Verification items for this drawing (mm, ordinates from the low corner). A direction names the side the tool comes from. Give positions to 0.01 mm unless a question says otherwise; leave off trailing zeros. Write each loop counter-clockwise with the first axis right and the second up, starting at its lowest first coordinate (ties: lowest second). Pieces come first, ordered by that corner, then holes. Notation, with made-up numbers: (49, 55.25) -> (65, 55.25) arc R27 cw to (65, 86.25) -> close; hole circle Ø6 at (20, 14.25). An arc over 180 degrees is marked (long way). Use one line per item in the form item = value. Start each with the question number.
(1) Section check A-A, the plane z = 19.25. Record the cut outline in (x, y).
(2) Section check B-B, the plane y = 9.75. Record the cut outline in (x, z).
(3) Section check C-C, the plane x = 4. Record the cut outline in (y, z), plus the area to 3 significant figures.
(4) Scan lines: L1, parallel to Z at x = 7, y = 0.5; L2, parallel to Z at x = 5.75, y = 12 (1 decimal); L3, parallel to Z at x = 7, y = 5.5. Record each from-to range of solid material in increasing order.
(5) Depth check by flat-ended pin: pin 1 Ø1 at (y, z) = (4, 7) entering from -X; pin 2 Ø7 at (x, y) = (6.57, 6.9) entering from +Z; pin 3 Ø6 at (y, z) = (10.5, 17) entering from -X. Enter the tip coordinate at first touch or a pass-through.
(6) Section check D-D, the plane y = 6.9. Record the cut outline in (x, z) (1 decimal).
(7) Set-up check for the marked faces 1, 2 and 3: record each of +Z, -Z, +X, -X, +Y, -Y from which the full face is reachable in a straight line by a thin tool's end or side.
(8) Release check for a two-part mould opening along Z. For the marked faces 4, 5 and 6 record: pulls with the +Z half, pulls with the -Z half, needs draft (parallel to the pull), parting line crosses it, or undercut.
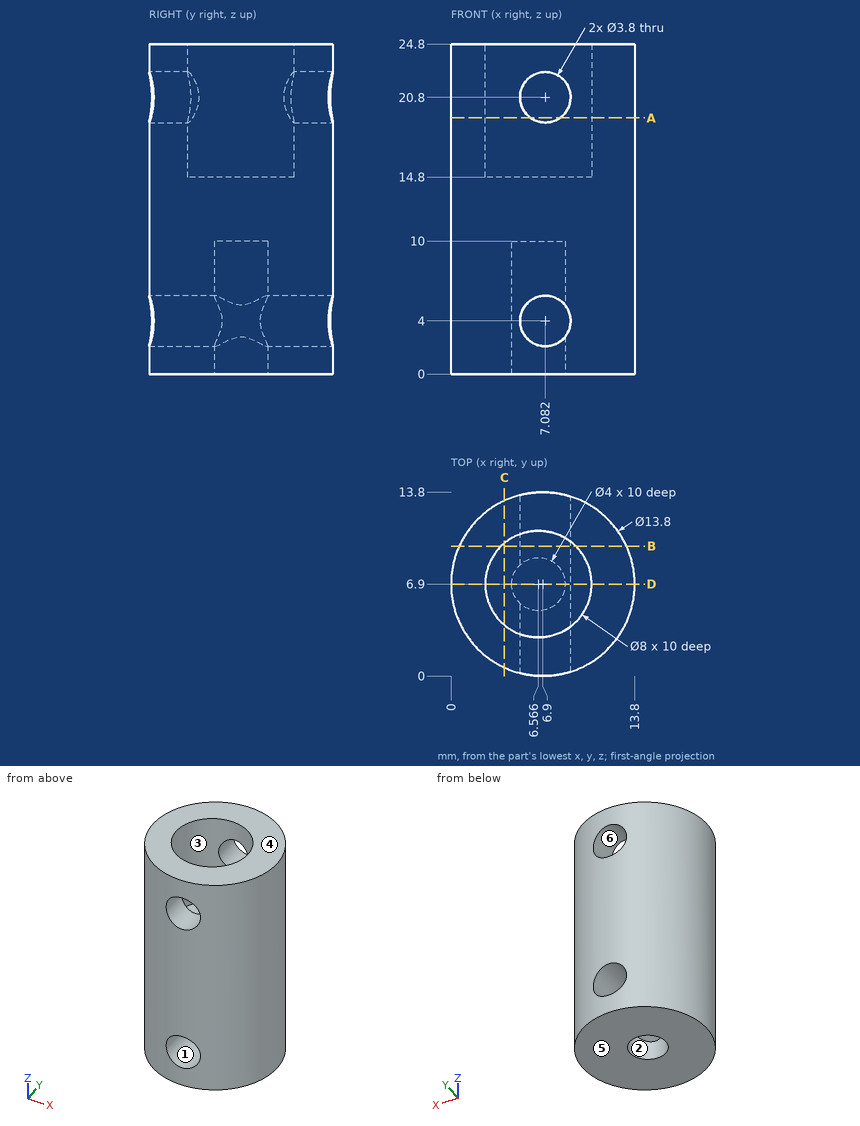
Completed:
q1.outline = (5.98, 0.06) -> (5.98, 2.94) arc R4 cw to (5.98, 10.86) -> (5.98, 13.74) arc R6.9 ccw to start; (8.18, 0.12) arc R6.9 ccw to (8.18, 13.68) -> (8.18, 10.56) arc R4 cw to (8.18, 3.24) -> close
q2.outline = (0.62, 0) -> (13.18, 0) -> (13.18, 24.8) -> (9.37, 24.8) -> (9.37, 14.8) -> (3.76, 14.8) -> (3.76, 24.8) -> (0.62, 24.8) -> close; hole circle Ø3.8 at (7.08, 4)
q3.outline = (0.64, 0) -> (13.16, 0) -> (13.16, 24.8) -> (9.97, 24.8) -> (9.97, 14.8) -> (3.83, 14.8) -> (3.83, 24.8) -> (0.64, 24.8) -> close
q3.area = 249 mm²
q4.L1 = 0 to 2.1, 5.9 to 18.9, 22.7 to 24.8
q4.L2 = 0 to 2.6, 5.4 to 19.4, 22.2 to 24.8
q4.L3 = 10 to 14.8
q5.pin_1 = 0.43
q5.pin_2 = 14.8
q5.pin_3 = 0.03
q6.outline = (0, 0) -> (4.6, 0) -> (4.6, 10) -> (8.6, 10) -> (8.6, 5.2) arc R1.9 cw to (8.6, 2.8) -> (8.6, 0) -> (13.8, 0) -> (13.8, 24.8) -> (10.6, 24.8) -> (10.6, 14.8) -> (2.6, 14.8) -> (2.6, 24.8) -> (0, 24.8) -> close
q7.face_1 = +Y, -Y
q7.face_2 = -Z
q7.face_3 = +Z
q8.face_4 = pulls with the +Z half
q8.face_5 = pulls with the -Z half
q8.face_6 = undercut
